```python
from build123d import *

# Parameters (mm, degrees)
SKETCH1_W           = 203.2
SKETCH1_H           = 127
BOSS_EXTRUDE1_DEPTH = 3.175
SKETCH2_W           = 25.4
SKETCH2_H           = 3.175
BOSS_EXTRUDE2_DEPTH = 3.175
SKETCH3_W           = 25.4
SKETCH3_H           = 3.175
BOSS_EXTRUDE3_DEPTH = 3.175
SKETCH4_W           = 25.908
SKETCH4_H           = 3.175
CUT_EXTRUDE1_DEPTH  = 3.175
SKETCH5_W           = 25.908
SKETCH5_H           = 3.175
CUT_EXTRUDE2_DEPTH  = 3.175
SKETCH7_W           = 26.67
SKETCH7_H           = 71.628
CUT_EXTRUDE3_DEPTH  = 3.175


with BuildPart() as part:
    # Sketch1 → Boss-Extrude1 (new body)
    with BuildSketch(Plane(origin=(0, 0, 0), x_dir=(1, 0, 0), z_dir=(0, 1, 0))):
        with Locations((94.089247312, -24.546505376)):
            Rectangle(SKETCH1_W, SKETCH1_H)
    extrude(amount=BOSS_EXTRUDE1_DEPTH)

    # Sketch2 → Boss-Extrude2 (add)
    with BuildSketch(Plane.XY.offset(88.046505376)):
        with Locations((119.489247312, 1.5875)):
            Rectangle(SKETCH2_W, SKETCH2_H)
        with Locations((30.589247312, 1.5875)):
            Rectangle(SKETCH2_W, SKETCH2_H)
    extrude(amount=BOSS_EXTRUDE2_DEPTH)

    # Sketch3 → Boss-Extrude3 (add)
    with BuildSketch(Plane(origin=(0, 0, -38.953494624), x_dir=(-1, 0, 0), z_dir=(0, 0, -1))):
        with Locations((-119.489247312, 1.5875)):
            Rectangle(SKETCH3_W, SKETCH3_H)
        with Locations((-30.589247312, 1.5875)):
            Rectangle(SKETCH3_W, SKETCH3_H)
    extrude(amount=BOSS_EXTRUDE3_DEPTH)

    # Sketch4 → Cut-Extrude1 (cut)
    with BuildSketch(Plane(origin=(195.689247312, 0, 0), x_dir=(0, 0, -1), z_dir=(1, 0, 0))):
        with Locations((-24.546505376, 1.5875)):
            Rectangle(SKETCH4_W, SKETCH4_H)
    extrude(amount=-CUT_EXTRUDE1_DEPTH, mode=Mode.SUBTRACT)

    # Sketch5 → Cut-Extrude2 (cut)
    with BuildSketch(Plane.ZY.offset(7.510752688)):
        with Locations((24.546505376, 1.5875)):
            Rectangle(SKETCH5_W, SKETCH5_H)
    extrude(amount=-CUT_EXTRUDE2_DEPTH, mode=Mode.SUBTRACT)

    # Sketch7 → Cut-Extrude3 (cut)
    with BuildSketch(Plane(origin=(0, 3.175, 0), x_dir=(1, 0, 0), z_dir=(0, 1, 0))):
        with Locations((94.089247312, -24.546505376)):
            Rectangle(SKETCH7_W, SKETCH7_H)
    extrude(amount=-CUT_EXTRUDE3_DEPTH, mode=Mode.SUBTRACT)


solid = part.part
```
Check sheet for the modelled part. Datum: model origin and axes. Units: mm. Round coordinates to 2 decimals unless told otherwise and drop trailing zeros. Loops run counter-clockwise (first coordinate to the right, second up) from the corner with the lowest first, then second, coordinate; pieces in that order, holes last. Notation, with made-up numbers: (32, 26) - (67, 26) arc R16 cw to (67, 41) - close; hole circle Ø10 at (72, -15). An arc over 180 degrees is marked (long way). Answer as a JSON object with one key per item and string values. Group by question number.
Q1. Scan lines: line 1 along X through (y, z) = (2, 10.5); line 2 along X through (y, z) = (0.5, 17.5); line 3 along Z through (x, y) = (4.5, 3). Record each from-to range of solid material in increasing order. Write a range as [from, to].
Q2. Sectioned sample at B-B, the plane x = 104.5. Enter the section's corners in (y, z) (1 decimal).
Q3. Gauge pin test, flat ends, axial feed: P1, Ø1.6, axis at x = 6, y = 1.5, coming from the -Z side; P2, Ø1.6, axis at y = 1.5, z = 35.5, coming from the -X side; P3, Ø1, axis at x = 99, y = 2, coming from the +Z side; P4, Ø2, axis at x = 83, z = 0, coming from the -Y side. Record the tip position at first contact, or that the pin passes through.
Q4. Sectioned sample at D-D, the plane x = 68. Enter the section's corners in (y, z) (1 decimal).
Q5. Mould release check, pull along Y, two halves, no side actions. Record for faces 1 (the face through (70, 3.175, 24)), 2 (the face through (70, 0, 24)): released by +Y, released by -Y, zero draft, split by the parting line, or undercut.
Q6. Sectioned sample at A-A, the plane z = 6. Enter the section's corners in (x, y) (3 decimals).
Solution:
{
 "1": {"line 1": "x = [-7.51, 80.75], [107.42, 195.69]", "line 2": "x = [-4.34, 80.75], [107.42, 192.51]", "line 3": "z = [-38.95, 88.05]"},
 "2": {"outline": "(0, -39) - (3.2, -39) - (3.2, -11.3) - (0, -11.3) - close; (0, 60.4) - (3.2, 60.4) - (3.2, 88) - (0, 88) - close"},
 "3": {"P1": "stops at z = -38.95", "P2": "stops at x = -4.34", "P3": "stops at z = 88.05", "P4": "passes through"},
 "4": {"outline": "(0, -39) - (3.2, -39) - (3.2, 88) - (0, 88) - close"},
 "5": {"face 1": "released by +Y", "face 2": "released by -Y"},
 "6": {"outline": "(-7.511, 0) - (80.754, 0) - (80.754, 3.175) - (-7.511, 3.175) - close; (107.424, 0) - (195.689, 0) - (195.689, 3.175) - (107.424, 3.175) - close"}
}
